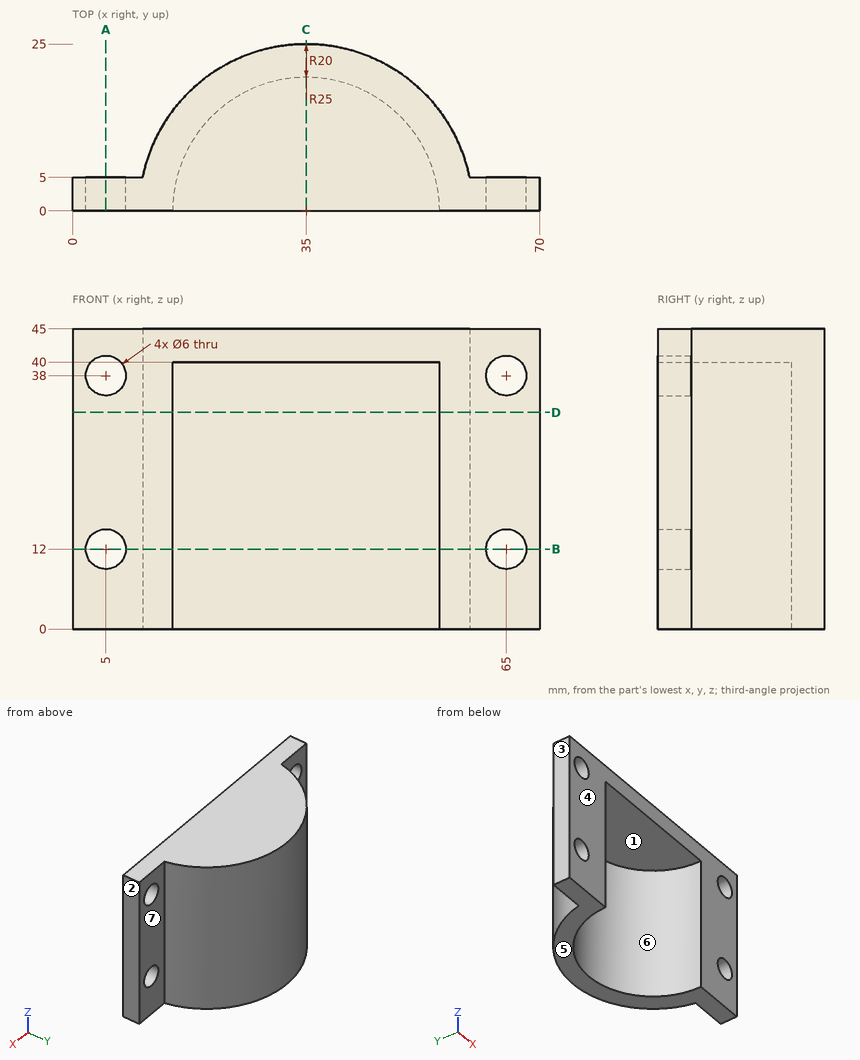
Source: three-view drawing plus pictorial views. Frame: mm from the lowest corner of the part. A direction names the side the tool comes from. Round coordinates to 2 decimals unless told otherwise and drop trailing zeros. Loops run counter-clockwise (first coordinate to the right, second up) from the corner with the lowest first, then second, coordinate; pieces in that order, holes last.
Q1. Section C-C, the plane x = 35. Return loops of the section in (y, z), plus the area to 3 significant figures.
Q2. First-contact query: P1, Ø8, axis at x = 5, z = 12, coming from the +Y side; P2, Ø11.5, axis at x = 7.5, z = 20.5, coming from the +Y side; P3, Ø1.5, axis at y = 11, z = 36.5, coming from the +X side. Flat tips, straight axial feed; report the tip coordinate or a pass-through.
Q3. Section A-A, the plane x = 5. Return loops of the section in (y, z).
Q4. Section B-B, the plane z = 12. Return loops of the section in (x, y).
Q5. Access query for the marked faces 5, 6 and 7. Directions: +Z, -Z, +X, -X, +Y, -Y. A direction counts if a zero-diameter tool reaches every point of the face in a straight line with its end or side. Return the directions, or none.
Q6. Mould query, pull axis X, two halves, no side actions, for the marked faces 1, 2, 3 and 4. Classes: pulls with the +X half, pulls with the -X half, needs draft (parallel to the pull), parting line crosses it, or undercut.
Q7. Ray query, line 1 (Z direction, x = 65, y = 3.6); line 2 (X direction, y = 2.85, z = 12); line 3 (X direction, y = 2.35, z = 38). Return the intervals inside material, ascending.
Q8. Section D-D, the plane z = 32.5. Return loops of the section in (x, y).
Solutions:
1. outline: (0, 40) - (20, 40) - (20, 0) - (25, 0) - (25, 45) - (0, 45) - close
1. area: 325 mm2
2. P1: stops at y = 5
2. P2: stops at y = 12.33
2. P3: stops at x = 57.8
3. outline: (0, 0) - (5, 0) - (5, 9) - (0, 9) - close; (0, 15) - (5, 15) - (5, 35) - (0, 35) - close; (0, 41) - (5, 41) - (5, 45) - (0, 45) - close
4. outline: (0, 0) - (2, 0) - (2, 5) - (0, 5) - close; (8, 0) - (15, 0) arc R20 cw to (55, 0) - (62, 0) - (62, 5) - (59.49, 5) arc R25 ccw to (10.51, 5) - (8, 5) - close; (68, 0) - (70, 0) - (70, 5) - (68, 5) - close
5. face 5: -Z, +X, -X, +Y, -Y
5. face 6: -Z, -Y
5. face 7: +Z, -Z, +X, +Y
6. face 1: undercut
6. face 2: pulls with the +X half
6. face 3: pulls with the -X half
6. face 4: needs draft
7. line 1: z = 0 to 9, 15 to 35, 41 to 45
7. line 2: x = 0 to 2, 8 to 15.2, 54.8 to 62, 68 to 70
7. line 3: x = 0 to 2, 8 to 15.14, 54.86 to 62, 68 to 70
8. outline: (0, 0) - (15, 0) arc R20 cw to (55, 0) - (70, 0) - (70, 5) - (59.49, 5) arc R25 ccw to (10.51, 5) - (0, 5) - close
